For this review, take the finished solid that the model builds, in its own axes (mm). A direction names the side the tool comes from. Round coordinates to 2 decimals unless told otherwise and drop trailing zeros. Loops run counter-clockwise (first coordinate to the right, second up) from the corner with the lowest first, then second, coordinate; pieces in that order, holes last.
1) Mouldability with a two-part tool opening along Z and no side actions: class faces 1 (the cylindrical face through (16.4, 2.96, 7.93)), 2 (the flat face through (22.5, 6, 0)), 3 (the cylindrical face through (-20.361, 5.916, 20.245)) as pulls with the +Z half, pulls with the -Z half, needs draft (parallel to the pull), parting line crosses it, or undercut.
2) Tool access review of faces 4 (the flat face through (3, 25, 4)), 5 (the cylindrical face through (10.354, 2.958, 10.455)), 6 (the cylindrical face through (-4.52, 39.53, 12.93)): name each direction out of +Z, -Z, +X, -X, +Y, -Y from which nothing blocks a thin tool from reaching the whole face with its end or side.
3) Insertion check: pin 1 (19 mm diameter, centred on y = 51.5, z = 18, fed in from +X); pin 2 (7.5 mm diameter, centred on x = 15, z = -15, fed in from +Y); pin 3 (10 mm diameter, centred on x = 17, z = -9, fed in from +Y); pin 4 (5.5 mm diameter, centred on x = 15, z = 15, fed in from +Y). Each pin has a flat end and moves straight along its axis. Give the tip position at first contact, or say it passes through.
4) Take a section at A-A (y = 51.5). State the section outline as (x, z) points, then the cut area to 3 significant figures.
5) Take a section at B-B (x = -13). State the section outline as (y, z) points, then the cut area to 3 significant figures.
6) Take a section at C-C (y = 25). State the section outline as (x, z) points, then the cut area to 3 significant figures.
7) Wall thickness on L1, parallel to X at y = 4.75, z = 15; L2, parallel to Z at x = -15, y = 8: over which ranges is each line inside the solid? List them lowest first.
8) Take a section at D-D (z = -10.5). State the section outline as (x, y) points, then the cut area to 3 significant figures.
```python
from build123d import *

# Parameters (mm, degrees)
SKETCH1_R                = 3.3
BOSS_EXTRUDE1_DEPTH      = 12
BOSS_EXTRUDE2_DEPTH      = 6
BOSS_EXTRUDE2_DEPTH_BACK = 6
CUT_EXTRUDE1_DEPTH       = 3
CUT_EXTRUDE2_DEPTH       = 3
CUT_EXTRUDE3_DEPTH       = 6
SKETCH7_R                = 5.5
CUT_EXTRUDE4_DEPTH       = 0.6
SKETCH8_R                = 5.5
CUT_EXTRUDE5_DEPTH       = 0.6
SKETCH9_R                = 5.5
CUT_EXTRUDE6_DEPTH       = 0.6
SKETCH10_R               = 5.5
CUT_EXTRUDE7_DEPTH       = 0.6


with BuildPart() as part:
    # Sketch1 → Boss-Extrude1 (new body)
    with BuildSketch(Plane(origin=(0, 0, 0), x_dir=(1, 0, 0), z_dir=(0, 1, 0))):
        with BuildLine():
            Line((-15, -22.5), (15, -22.5))
            ThreePointArc((15, -22.5), (20.303300859, -20.303300859), (22.5, -15))
            Line((22.5, -15), (22.5, 15))
            ThreePointArc((22.5, 15), (20.303300859, 20.303300859), (15, 22.5))
            Line((15, 22.5), (-15, 22.5))
            ThreePointArc((-15, 22.5), (-20.303300859, 20.303300859), (-22.5, 15))
            Line((-22.5, 15), (-22.5, -15))
            ThreePointArc((-22.5, -15), (-20.303300859, -20.303300859), (-15, -22.5))
        make_face()
        with Locations((15, 15)):
            Circle(SKETCH1_R, mode=Mode.SUBTRACT)
        with Locations((15, -15)):
            Circle(SKETCH1_R, mode=Mode.SUBTRACT)
        with Locations((-15, 15)):
            Circle(SKETCH1_R, mode=Mode.SUBTRACT)
        with Locations((-15, -15)):
            Circle(SKETCH1_R, mode=Mode.SUBTRACT)
    extrude(amount=BOSS_EXTRUDE1_DEPTH)

    # Sketch2 → Boss-Extrude2 (add, two sides)
    with BuildSketch(Plane(origin=(0, 0, 0), x_dir=(0, 0, -1), z_dir=(1, 0, 0))) as boss_extrude2_sk:
        with BuildLine():
            Line((-30.687542875, 48.666935264), (-22.5, 12))
            Line((-22.5, 12), (22.5, 12))
            Line((22.5, 12), (-7.027549789, 58.471752748))
            ThreePointArc((-7.027549789, 58.471752748), (-13.023153892, 39.49037874), (-30.687542875, 48.666935264))
        make_face()
    extrude(amount=BOSS_EXTRUDE2_DEPTH)
    extrude(boss_extrude2_sk.sketch, amount=-BOSS_EXTRUDE2_DEPTH_BACK)

    # Sketch3 → Cut-Extrude1 (cut)
    with BuildSketch(Plane(origin=(6, 0, 0), x_dir=(0, 0, -1), z_dir=(1, 0, 0))):
        with BuildLine():
            Line((-22.278487974, 36.245671412), (-17.213816554, 13.564143887))
            ThreePointArc((-17.213816554, 13.564143887), (-16.512544263, 12.439277054), (-15.261886881, 12))
            Line((-15.261886881, 12), (12.343334592, 12))
            ThreePointArc((12.343334592, 12), (14.096211469, 13.036972143), (14.031403855, 15.072577346))
            Line((14.031403855, 15.072577346), (-4.185678595, 43.743420591))
            ThreePointArc((-4.185678595, 43.743420591), (-5.810453328, 44.669841445), (-7.490581477, 43.848064146))
            ThreePointArc((-7.490581477, 43.848064146), (-13.023153892, 39.49037874), (-20.016350528, 38.657323856))
            ThreePointArc((-20.016350528, 38.657323856), (-21.785266488, 38.049800314), (-22.278487974, 36.245671412))
        make_face()
    extrude(amount=-CUT_EXTRUDE1_DEPTH, mode=Mode.SUBTRACT)

    # Sketch4 → Cut-Extrude2 (cut)
    with BuildSketch(Plane(origin=(-6, 0, 0), x_dir=(0, 0, -1), z_dir=(1, 0, 0))):
        with BuildLine():
            Line((-22.278487974, 36.245671412), (-17.213816554, 13.564143887))
            ThreePointArc((-17.213816554, 13.564143887), (-16.512544263, 12.439277054), (-15.261886881, 12))
            Line((-15.261886881, 12), (12.343334592, 12))
            ThreePointArc((12.343334592, 12), (14.096211469, 13.036972143), (14.031403855, 15.072577346))
            Line((14.031403855, 15.072577346), (-4.185678595, 43.743420591))
            ThreePointArc((-4.185678595, 43.743420591), (-5.810453328, 44.669841445), (-7.490581477, 43.848064146))
            ThreePointArc((-7.490581477, 43.848064146), (-13.023153892, 39.49037874), (-20.016350528, 38.657323856))
            ThreePointArc((-20.016350528, 38.657323856), (-21.785266488, 38.049800314), (-22.278487974, 36.245671412))
        make_face()
    extrude(amount=CUT_EXTRUDE2_DEPTH, mode=Mode.SUBTRACT)

    # Sketch5 → Revolve1 (revolve)
    with BuildSketch(Plane.XY.offset(18)):
        with BuildLine():
            Line((-7, 63.5), (-7, 57.5))
            Line((-7, 57.5), (7, 57.5))
            Line((7, 57.5), (7, 63.5))
            ThreePointArc((7, 63.5), (6.707106781, 64.207106781), (6, 64.5))
            Line((6, 64.5), (-6, 64.5))
            ThreePointArc((-6, 64.5), (-6.707106781, 64.207106781), (-7, 63.5))
        make_face()
    revolve(axis=Axis((7, 51.5, 18), (-1, 0, 0)))

    # Sketch6 → Cut-Extrude3 (cut)
    with BuildSketch(Plane(origin=(0, 0, 0), x_dir=(1, 0, 0), z_dir=(0, 1, 0))):
        with BuildLine():
            Line((-17, 6.5), (-17, -6.5))
            ThreePointArc((-17, -6.5), (-16.414213562, -7.914213562), (-15, -8.5))
            ThreePointArc((-15, -8.5), (-10.403805922, -10.403805922), (-8.5, -15))
            ThreePointArc((-8.5, -15), (-7.914213562, -16.414213562), (-6.5, -17))
            Line((-6.5, -17), (6.5, -17))
            ThreePointArc((6.5, -17), (7.914213562, -16.414213562), (8.5, -15))
            ThreePointArc((8.5, -15), (10.403805922, -10.403805922), (15, -8.5))
            ThreePointArc((15, -8.5), (16.414213562, -7.914213562), (17, -6.5))
            Line((17, -6.5), (17, 6.5))
            ThreePointArc((17, 6.5), (16.414213562, 7.914213562), (15, 8.5))
            ThreePointArc((15, 8.5), (10.403805922, 10.403805922), (8.5, 15))
            ThreePointArc((8.5, 15), (7.914213562, 16.414213562), (6.5, 17))
            Line((6.5, 17), (-6.5, 17))
            ThreePointArc((-6.5, 17), (-7.914213562, 16.414213562), (-8.5, 15))
            ThreePointArc((-8.5, 15), (-10.403805922, 10.403805922), (-15, 8.5))
            ThreePointArc((-15, 8.5), (-16.414213562, 7.914213562), (-17, 6.5))
        make_face()
    extrude(amount=CUT_EXTRUDE3_DEPTH, mode=Mode.SUBTRACT)

    # Sketch7 → Cut-Extrude4 (cut)
    with BuildSketch(Plane(origin=(0, 12, 0), x_dir=(1, 0, 0), z_dir=(0, 1, 0))):
        with Locations((15, 15)):
            Circle(SKETCH7_R)
    extrude(amount=-CUT_EXTRUDE4_DEPTH, mode=Mode.SUBTRACT)

    # Sketch8 → Cut-Extrude5 (cut)
    with BuildSketch(Plane(origin=(0, 12, 0), x_dir=(1, 0, 0), z_dir=(0, 1, 0))):
        with Locations((-15, 15)):
            Circle(SKETCH8_R)
    extrude(amount=-CUT_EXTRUDE5_DEPTH, mode=Mode.SUBTRACT)

    # Sketch9 → Cut-Extrude6 (cut)
    with BuildSketch(Plane(origin=(0, 12, 0), x_dir=(1, 0, 0), z_dir=(0, 1, 0))):
        with Locations((15, -15)):
            Circle(SKETCH9_R)
    extrude(amount=-CUT_EXTRUDE6_DEPTH, mode=Mode.SUBTRACT)

    # Sketch10 → Cut-Extrude7 (cut)
    with BuildSketch(Plane(origin=(0, 12, 0), x_dir=(1, 0, 0), z_dir=(0, 1, 0))):
        with Locations((-15, -15)):
            Circle(SKETCH10_R)
    extrude(amount=-CUT_EXTRUDE7_DEPTH, mode=Mode.SUBTRACT)


solid = part.part
```
Response:
1. face 1: undercut
1. face 2: needs draft
1. face 3: pulls with the +Z half
2. face 4: +X
2. face 5: -Y
2. face 6: -X
3. pin 1: stops at x = 7
3. pin 2: stops at y = 11.4
3. pin 3: stops at y = 12
3. pin 4: passes through
4. outline: (-7, 6) arc R1 ccw to (-6, 5) - (-6, 2.6) - (6, 2.6) - (6, 5) arc R1 ccw to (7, 6) - (7, 12) - (-7, 12) - close; (-7, 24) - (7, 24) - (7, 30) arc R1 ccw to (6, 31) - (-6, 31) arc R1 ccw to (-7, 30) - close
4. area: 224 mm2
5. outline: (0, -22.5) - (12, -22.5) - (12, -20.12) - (11.4, -20.12) - (11.4, -17.62) - (0, -17.62) - close; (0, -12.38) - (11.4, -12.38) - (11.4, -9.88) - (12, -9.88) - (12, 9.88) - (11.4, 9.88) - (11.4, 12.38) - (0, 12.38) - (0, 8.82) - (6, 8.82) - (6, -8.82) - (0, -8.82) - close; (0, 17.62) - (11.4, 17.62) - (11.4, 20.12) - (12, 20.12) - (12, 22.5) - (0, 22.5) - close
5. area: 302 mm2
6. outline: (-6, -14.24) - (6, -14.24) - (6, -7.72) - (3, -7.72) - (3, 19.77) - (6, 19.77) - (6, 25.4) - (-6, 25.4) - (-6, 19.77) - (-3, 19.77) - (-3, -7.72) - (-6, -7.72) - close
6. area: 311 mm2
7. L1: x = -22.5 to -18.3, -11.7 to -8.5, 8.5 to 11.7, 18.3 to 22.5
7. L2: z = -22.5 to -18.3, -11.7 to 11.7, 18.3 to 22.5
8. outline: (-22.5, 0) - (-10.31, 0) - (-10.31, 6) - (10.31, 6) - (10.31, 0) - (22.5, 0) - (22.5, 12) - (18.16, 12) - (18.16, 11.4) - (11.84, 11.4) - (11.84, 12) - (3, 12) - (3, 20.63) - (6, 20.63) - (6, 30.89) - (-6, 30.89) - (-6, 20.63) - (-3, 20.63) - (-3, 12) - (-11.84, 12) - (-11.84, 11.4) - (-18.16, 11.4) - (-18.16, 12) - (-22.5, 12) - close
8. area: 584 mm2
